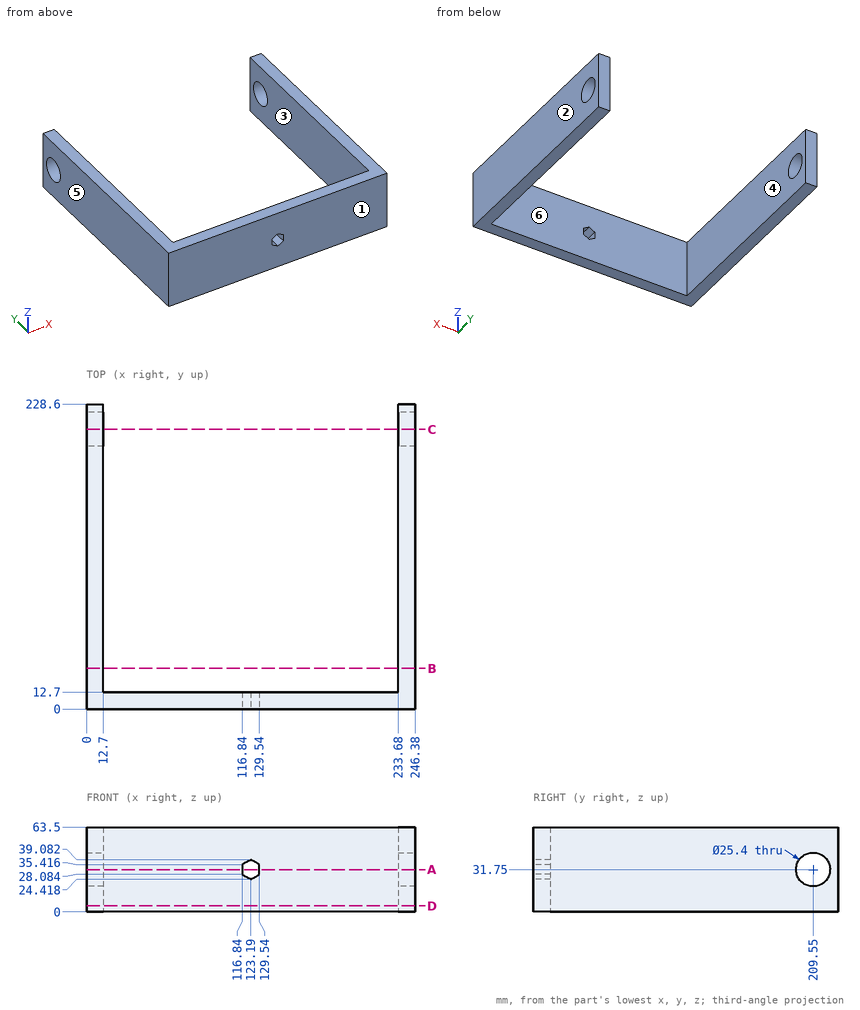
Can you work these out from the drawing? Everything is in mm from the part's minimum corner. A direction names the side the tool comes from. Coordinates: 2 decimals unless noted, no trailing zeros. Loops run counter-clockwise (first coordinate to the right, second up) from the corner with the lowest first, then second, coordinate; pieces in that order, holes last.
1) Imagine slicing it at D-D on z = 4.5. List the corners of the cut face in (x, y) for me, plus the area to 3 significant figures.
2) For pin 1 (4 mm diameter, centred on x = 92.5, z = 53.5, fed in from +Y), with a flat end and sliding along its axis, tell me the tip position at first contact or that it passes through.
3) Imagine slicing it at A-A on z = 31.75. List the corners of the cut face in (x, y) for me.
4) Imagine slicing it at B-B on y = 30.5. List the corners of the cut face in (x, z) for me.
5) I need wall thicknesses on probe 1 along X at (y, z) = (32.5, 45.5); probe 2 along Z at (x, y) = (243, 209); probe 3 along Y at (x, z) = (5.75, 31.75). Which ranges of each line are inside material? Lowest first, please.
6) Imagine slicing it at C-C on y = 209.55. List the corners of the cut face in (x, z) for me.
7) Which directions (+Z, -Z, +X, -X, +Y, -Y) give clear straight access to the entire face, cutting with the end or side of a thin tool? Please do the marked faces 5 and 6.
8) Thinking about a two-plate mould opening in X: for the marked faces 1, 2, 3 and 4, which applies, pulls with the +X half, pulls with the -X half, needs draft (parallel to the pull), parting line crosses it, or undercut?
Completed:
1. outline: (0, 0) - (246.38, 0) - (246.38, 228.6) - (233.68, 228.6) - (233.68, 12.7) - (12.7, 12.7) - (12.7, 228.6) - (0, 228.6) - close
1. area: 8,610 mm2
2. pin 1: stops at y = 12.7
3. outline: (0, 0) - (116.84, 0) - (116.84, 12.7) - (12.7, 12.7) - (12.7, 196.85) - (0, 196.85) - close; (0, 222.25) - (12.7, 222.25) - (12.7, 228.6) - (0, 228.6) - close; (129.54, 0) - (246.38, 0) - (246.38, 196.85) - (233.68, 196.85) - (233.68, 12.7) - (129.54, 12.7) - close; (233.68, 222.25) - (246.38, 222.25) - (246.38, 228.6) - (233.68, 228.6) - close
4. outline: (0, 0) - (12.7, 0) - (12.7, 63.5) - (0, 63.5) - close; (233.68, 0) - (246.38, 0) - (246.38, 63.5) - (233.68, 63.5) - close
5. probe 1: x = 0 to 12.7, 233.68 to 246.38
5. probe 2: z = 0 to 19.06, 44.44 to 63.5
5. probe 3: y = 0 to 196.85, 222.25 to 228.6
6. outline: (0, 0) - (12.7, 0) - (12.7, 19.05) - (0, 19.05) - close; (0, 44.45) - (12.7, 44.45) - (12.7, 63.5) - (0, 63.5) - close; (233.68, 0) - (246.38, 0) - (246.38, 19.05) - (233.68, 19.05) - close; (233.68, 44.45) - (246.38, 44.45) - (246.38, 63.5) - (233.68, 63.5) - close
7. face 5: +Z, -Z, -X, +Y, -Y
7. face 6: +Z, -Z, +Y
8. face 1: needs draft
8. face 2: pulls with the +X half
8. face 3: undercut
8. face 4: undercut
